```python
from build123d import *

# Parameters (mm, degrees)
HEXAGONO_DEPTH      = 5.2
TALADRO_PROFILE_R   = 2.45875
ROSCA_M6X1_0_PITCH  = 1
ROSCA_M6X1_0_HEIGHT = 5.2
ROSCA_M6X1_0_RADIUS = 2.4587


with BuildPart() as part:
    # Sk_Hexagono → Hexagono (new body)
    with BuildSketch(Plane(origin=(0, 0, 0), x_dir=(1, 0, 0), z_dir=(0, 1, 0))):
        Polygon((5, -2.886751346), (0, -5.773502692), (-5, -2.886751346), (-5, 2.886751346), (0, 5.773502692), (5, 2.886751346), align=None)
    extrude(amount=HEXAGONO_DEPTH)

    # Taladro: sweep along a curve in space
    with BuildLine() as taladro_path:
        Line((0, -1, 0), (0, 6.2, 0))
    # Taladro profile (on start of the path) → Taladro (sweep, cut)
    with BuildSketch(Plane.ZX.offset(-1)):
        Circle(TALADRO_PROFILE_R)
    sweep(path=taladro_path.line, mode=Mode.SUBTRACT)

    # Rosca_M6x1,0: sweep along a helix
    with BuildLine() as rosca_m6x1_0_path:
        Helix(ROSCA_M6X1_0_PITCH, ROSCA_M6X1_0_HEIGHT, ROSCA_M6X1_0_RADIUS, center=(0, 0, 0), direction=(0, 1, 0), lefthand=True)
    # Sk_Perfil_rosca → Rosca_M6x1,0 (sweep, cut)
    with BuildSketch(Plane(origin=(0, 0, 0), x_dir=(0, 0, -1), z_dir=(1, 0, 0))):
        Polygon((-2.2587, -0.6), (-3.0721, 0), (-2.2587, 0.6), align=None)
    sweep(path=rosca_m6x1_0_path.line, is_frenet=True, mode=Mode.SUBTRACT)


solid = part.part
```
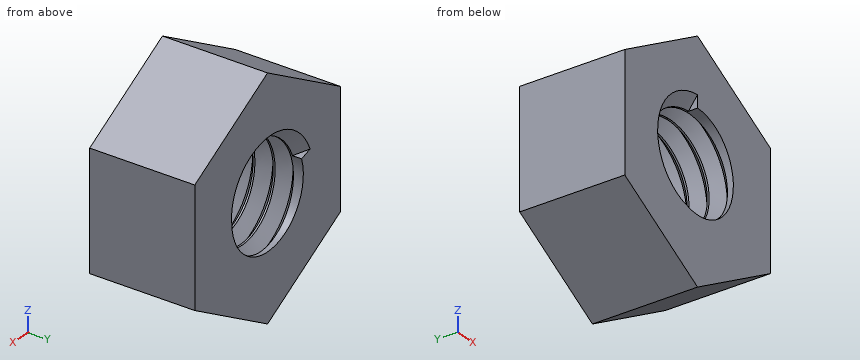
The model under review builds one solid part; all positions refer to its coordinate system, in mm. Round coordinates to 2 decimals unless told otherwise and drop trailing zeros. Loops run counter-clockwise (first coordinate to the right, second up) from the corner with the lowest first, then second, coordinate; pieces in that order, holes last. Notation, with made-up numbers: M 83,21.5 L 141,21.5 A21 cw 141,60.5 Z; hole C 71,20 d2. An arc over 180 degrees is marked long. Write item = value, one per line.
Item 1: Take a section at B-B on x = 4.5. Write out the cut boundary in (y, z), then the cut area to 3 significant figures.
Return value:
outline = M 0,-3.18 L 5.2,-3.18 L 5.2,3.18 L 0,3.18 Z
area = 33.0 mm2
Item 2: For line 1 (X direction, y = 4.85, z = 1); line 2 (X direction, y = 4, z = -0.75); line 3 (X direction, y = 4.2, z = -4), list the stretches that pass through material, from the lowest coordinate up. Write a range as [from, to].
Return value:
line_1 = [-5, -2.42], [2.84, 5]
line_2 = [-5, -2.56], [2.56, 5]
line_3 = [-3.07, 3.07]
Item 3: Insertion check: P1, Ø5.5, axis at x = 0, z = 0, coming from the +Y side. The pin has a flat end and moves straight along its axis. Give the tip position at first contact, or say it passes through.
Return value:
P1 = 5.2
Item 4: Take a section at A-A on z = -4. Write out the cut boundary in (x, y), then the cut area to 3 significant figures.
Return value:
outline = M -3.07,0 L 3.07,0 L 3.07,5.2 L -3.07,5.2 Z
area = 31.9 mm2
